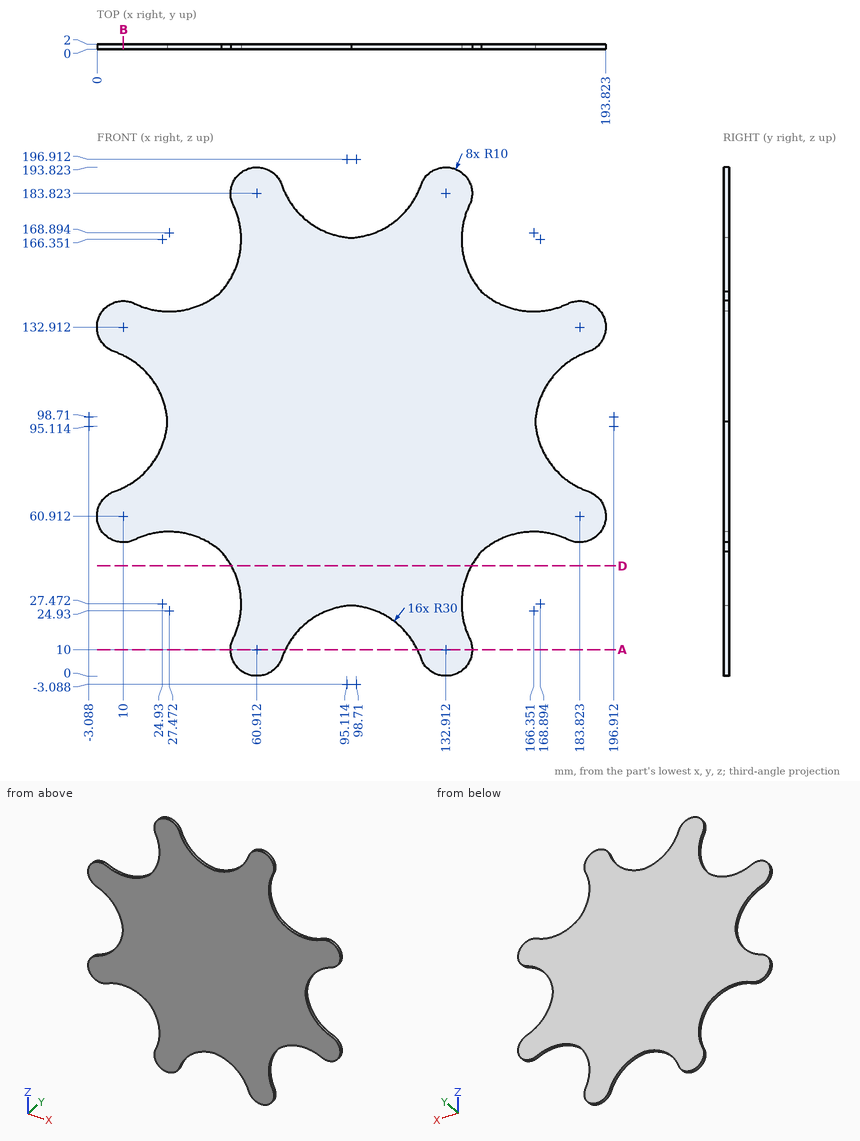
The drawing under review shows one solid part. Ordinate dimensions are in mm from its lowest x, y, z. Give positions to 0.01 mm unless a question says otherwise; leave off trailing zeros. Write each loop counter-clockwise with the first axis right and the second up, starting at its lowest first coordinate (ties: lowest second). Pieces come first, ordered by that corner, then holes.
1. Wall thickness on L1, parallel to X at y = 0.3, z = 174 (1 decimal); L2, parallel to Z at x = 19, y = 1.8 (1 decimal); L3, parallel to X at y = 0.4, z = 21 (1 decimal): over which ranges is each line inside the solid? List them lowest first.
2. Add section A-A, the plane z = 10. Write out the cut boundary in (x, y) (1 decimal).
3. For P1, Ø1.5, axis at x = 36, z = 80, coming from the -Y side, flat-tipped, find the tip position at first contact; note if it passes through.
4. Add section D-D, the plane z = 42. Write out the cut boundary in (x, y), plus the area to 3 significant figures.
5. Add section B-B, the plane x = 10. Write out the cut boundary in (y, z) (1 decimal).
Worked answers:
1. L1: x = 53.9 to 79.3, 114.5 to 139.9
1. L2: z = 53.7 to 78.4, 115.4 to 140.1
1. L3: x = 54.2 to 80.8, 113 to 139.6
2. outline: (50.9, 0) - (71.7, 0) - (71.7, 2) - (50.9, 2) - close; (122.1, 0) - (142.9, 0) - (142.9, 2) - (122.1, 2) - close
3. P1: stops at y = 0
4. outline: (51.18, 0) - (142.65, 0) - (142.65, 2) - (51.18, 2) - close
4. area: 183 mm2
5. outline: (0, 50.9) - (2, 50.9) - (2, 71.7) - (0, 71.7) - close; (0, 122.1) - (2, 122.1) - (2, 142.9) - (0, 142.9) - close
